Answer from the drawing. Dimensions are ordinates in mm from the lowest x, y and z of the part. A direction names the side the tool comes from. Coordinates: 2 decimals unless noted, no trailing zeros. Loops run counter-clockwise (first coordinate to the right, second up) from the corner with the lowest first, then second, coordinate; pieces in that order, holes last.
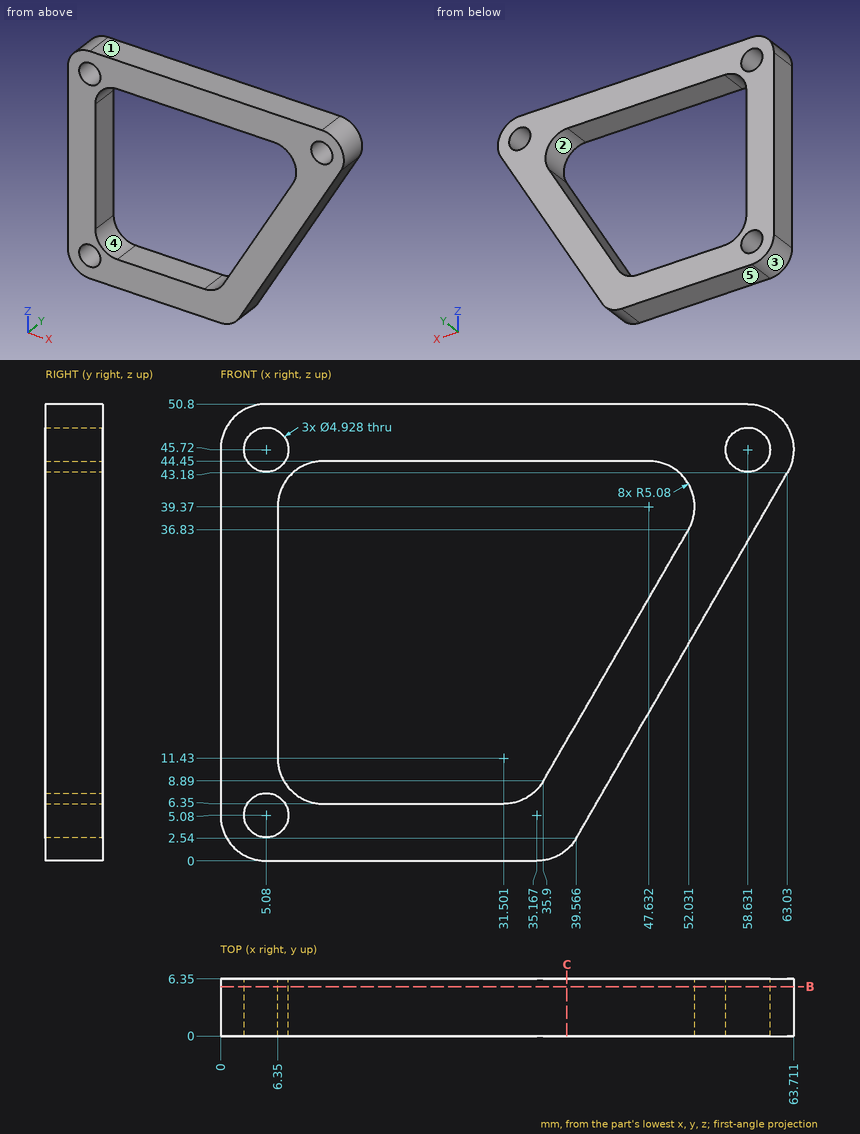
Item 1: Which of the six approach directions +Z, -Z, +X, -X, +Y, -Y give full straight-line access (tool end or side, diameter ignored) to the marked faces 4 and 5?
Numbers:
face 4: +Y, -Y
face 5: -Z, +X, -X, +Y, -Y
Item 2: Find the intervals of material crossed by line 1 along Z through (x, y) = (5.08, 1.75); line 2 along Z through (x, y) = (13, 0.5); line 3 along X through (y, z) = (5, 9) (1 decimal), in increasing order.
Numbers:
line 1: z = 0 to 2.62, 7.54 to 43.26, 48.18 to 50.8
line 2: z = 0 to 6.35, 44.45 to 50.8
line 3: x = 0 to 7, 36 to 43.3
Item 3: Given pin 1 (6.5 mm diameter, centred on x = 5.08, z = 45.72, fed in from -Y); pin 2 (3 mm diameter, centred on x = 58.63, z = 45.72, fed in from +Y); pin 3 (1.5 mm diameter, centred on x = 55.5, y = 4.5, fed in from -Z); pin 4 (2 mm diameter, centred on x = 50.5, y = 1, fed in from -Z) (1 decimal), each flat-ended and moving along its own axis, determine where each tip first touches the part or whether it passes through.
Numbers:
pin 1: stops at y = 0
pin 2: passes through
pin 3: stops at z = 28.84
pin 4: stops at z = 19.7
Item 4: A cutting plane is placed at B-B on y = 5.5. Determine the outline of the cut face in (x, z), then the cut area to 3 significant figures.
Numbers:
outline: (0, 5.08) arc R5.08 ccw to (5.08, 0) - (35.17, 0) arc R5.08 ccw to (39.57, 2.54) - (63.03, 43.18) arc R5.08 ccw to (58.63, 50.8) - (5.08, 50.8) arc R5.08 ccw to (0, 45.72) - close; hole circle Ø4.93 at (5.08, 5.08); hole circle Ø4.93 at (5.08, 45.72); hole (6.35, 11.43) arc R5.08 ccw to (11.43, 6.35) - (31.5, 6.35) arc R5.08 ccw to (35.9, 8.89) - (52.03, 36.83) arc R5.08 ccw to (47.63, 44.45) - (11.43, 44.45) arc R5.08 ccw to (6.35, 39.37) - close; hole circle Ø4.93 at (58.63, 45.72)
area: 1,130 mm2
Item 5: Determine the mould class of the marked faces 1, 2 and 3 for opening direction X: released by +X, released by -X, zero draft, split by the parting line, or undercut.
Numbers:
face 1: zero draft
face 2: undercut
face 3: released by -X
Item 6: A cutting plane is placed at C-C on x = 38.5. Determine the outline of the cut face in (y, z).
Numbers:
outline: (0, 1.25) - (6.35, 1.25) - (6.35, 13.39) - (0, 13.39) - close; (0, 44.45) - (6.35, 44.45) - (6.35, 50.8) - (0, 50.8) - close
